Autodesk Inventor part; units mm, degrees
ref_plane "YZ Plane" through (0, 0, 0) normal (1, 0, 0) x (0, 1, 0)
ref_plane "XZ Plane" through (0, 0, 0) normal (0, 1, 0) x (-1, 0, 0)
ref_plane "XY Plane" through (0, 0, 0) normal (0, 0, 1) x (1, 0, 0)
sketch "スケッチ1" plane through (0, 0, 0) normal (0, 0, 1) x (1, 0, 0)
  line L0 (-12.5, -12.5) -> (12.5, -12.5) construction
  line L1 (12.5, -12.5) -> (12.5, 12.5) construction
  line L2 (12.5, 12.5) -> (-12.5, 12.5) construction
  line L3 (-12.5, 12.5) -> (-12.5, -12.5) construction
  line L4 (-12.5, -12.5) -> (12.5, 12.5) construction
  line L5 (12.5, -12.5) -> (-12.5, 12.5) construction
  line L6 (-8.1, 12.5) -> (-12.5, 12.5)
  line L7 (-12.5, 12.5) -> (-12.5, 8.1)
  line L8 (8.1, 12.5) -> (12.5, 12.5)
  line L9 (12.5, 12.5) -> (12.5, 8.1)
  line L10 (-12.5, -8.1) -> (-12.5, -12.5)
  line L11 (-12.5, -12.5) -> (-8.1, -12.5)
  line L12 (8.1, -12.5) -> (12.5, -12.5)
  line L13 (12.5, -12.5) -> (12.5, -8.1)
  line L14 (-6, 12.5) -> (-6, 14.5)
  line L15 (-6, 14.5) -> (6, 14.5)
  line L16 (6, 14.5) -> (6, 12.5)
  arc A0 (-8.1, 12.5) -> (-6, 12.5) centre (-7.05, 12.5) ccw
  arc A1 (6, 12.5) -> (8.1, 12.5) centre (7.05, 12.5) ccw
  line L17 (0, 12.5) -> (0, 0) construction
  line L18 (0, 0) -> (12.5, 0) construction
  line L19 (-12.5, 6) -> (-14.5, 6) construction
  line L20 (-14.5, 6) -> (-14.5, -6) construction
  line L21 (-14.5, -6) -> (-12.5, -6) construction
  arc A2 (-12.5, 6) -> (-12.5, 8.1) centre (-12.5, 7.05) ccw
  arc A3 (-12.5, -8.1) -> (-12.5, -6) centre (-12.5, -7.05) ccw construction
  line L22 (-6, -12.5) -> (-6, -14.5)
  line L23 (-6, -14.5) -> (6, -14.5)
  line L24 (6, -14.5) -> (6, -12.5)
  arc A4 (-6, -12.5) -> (-8.1, -12.5) centre (-7.05, -12.5) ccw
  arc A5 (8.1, -12.5) -> (6, -12.5) centre (7.05, -12.5) ccw
  line L25 (12.5, 6) -> (14.5, 6) construction
  line L26 (14.5, 6) -> (14.5, -6) construction
  line L27 (14.5, -6) -> (12.5, -6) construction
  arc A6 (12.5, 8.1) -> (12.5, 6) centre (12.5, 7.05) ccw construction
  arc A7 (12.5, -6) -> (12.5, -8.1) centre (12.5, -7.05) ccw construction
  line L28 (-9.05, 12.5) -> (-5.95, 12.5) construction
  line L29 (-5.95, 12.5) -> (-5.95, 9.5) construction
  line L30 (-5.95, 9.5) -> (-9.05, 9.5) construction
  line L31 (-9.05, 9.5) -> (-9.05, 12.5) construction
  line L32 (-12.5, 9.05) -> (-9.5, 9.05) construction
  line L33 (-9.5, 5.95) -> (-12.5, 5.95) construction
  line L34 (-12.5, 5.95) -> (-12.5, 9.05) construction
  line L35 (-7.5, 12.5) -> (-7.5, 9.5) construction
  line L36 (-9.5, 7.5) -> (-12.5, 7.5) construction
  line L37 (-12.5, -12.5) -> (-12.5, 12.5)
  line L38 (12.5, -12.5) -> (12.5, 12.5)
  dimension "d0" = 25
  dimension "d1" = 1.05
  dimension "d2" = 2
  dimension "d3" = 6.5
  dimension "d4" = 3.1
  dimension "d6" = 3
  dimension "d17" = 5
  dimension "d18" = 5
  dimension "d46" = 25
extrude "押し出し1" add sketch "スケッチ1" along normal blind 4
mirror "ミラー1" about plane through (0, 0, 0) normal (0, 0, -1) of "押し出し1"
sketch "スケッチ2" plane through (-12.5, -12.5, 4) normal (0, -1, 0) x (1, 0, 0)
  line L0 (6.5, 0) -> (18.5, 0) construction
  line L1 (12.5, 0) -> (12.5, -5) construction
  line L2 (0, -8) -> (0, 0) construction
  line L3 (0, -2.5) -> (22.3, -2.5) construction
  point P0 (12.5, -4)
  point P1 (2.7, -2.5)
  point P2 (0.0223, -2.5)
  dimension "d52" = 2.7
  dimension "d53" = 2.5
hole "穴1" at (-9.8, -12.5, 1.5) at (9.8, -12.5, 1.5) direction (0, 1, 0) diameter 2.459 depth 8.8
pattern_circular "円形状パターン1" count 2 over 360 about axis through (0, 0, -10) along (0, 0, 1) of "穴1"
sketch "スケッチ4" plane through (-8.1, -12.5, -4) normal (0, 0, -1) x (-1, 0, 0)
  circle A0 centre (-8.1, 4) radius 1.5
  line L0 (-8.1, 4) -> (-8.1, 12.5) construction
  circle A1 centre (0.4, 12.5) radius 1.5
  circle A2 centre (-8.1, 21) radius 1.5
  circle A3 centre (-16.6, 12.5) radius 1.5
  dimension "d35" = 3
  dimension "d36" = 8.5
  dimension "d39" = 360
extrude "押し出し3" cut sketch "スケッチ4" against normal through all
sketch "スケッチ5" plane through (-8.1, -12.5, -4) normal (0, 0, -1) x (-1, 0, 0)
  circle A0 centre (-8.1, 12.5) radius 5.05
  dimension "d43" = 10.1
extrude "押し出し4" cut sketch "スケッチ5" against normal blind 2
sketch "スケッチ6" plane through (0, 0, 4) normal (0, 0, 1) x (1, 0, 0)
  circle A0 centre (8.5, 0) radius 1.5 construction
  circle A1 centre (0, 8.5) radius 1.5 construction
  circle A2 centre (-8.5, 0) radius 1.5 construction
  circle A3 centre (0, -8.5) radius 1.5 construction
  line L0 (0, -8.5) -> (0, 8.5) construction
  line L1 (8.5, 0) -> (-8.5, 0) construction
  circle A4 centre (0, 0) radius 5.05
  dimension "d47" = 10.1
extrude "押し出し5" cut sketch "スケッチ6" against normal up to surface (8 mm away)
sketch "スケッチ8" plane through (6, 14.5, -4) normal (0, 0, -1) x (-1, 0, 0)
  line L0 (0, -29) -> (0, -27)
  line L1 (12, -29) -> (0, -29)
  line L2 (12, -27) -> (12, -29)
  line L3 (0, 0) -> (12, 0)
  line L4 (0, -2) -> (0, 0)
  line L5 (12, 0) -> (12, -2)
  line L6 (0, -27) -> (12, -27)
  line L7 (0, -2) -> (12, -2)
  point P0 (6, -14.5)
extrude "押し出し6" cut sketch "スケッチ8" against normal blind 3
equation "\"d18\" = d17"
properties part number "頭_サーボホーンフレーム" material "アセタール樹脂、黒"
Design review of the part built by this model. Coordinates are the model's own, in mm. A direction names the side the tool comes from. Coordinates: 2 decimals unless noted, no trailing zeros. Order: outer loops, then holes, each group sorted by start corner. A loop starts at its lowest first (then second) coordinate and runs counter-clockwise, first axis right, second up.
Item 1: The part is to be moulded in two halves that separate along Z. For faces 4 (the flat face through (-10, 3.7, 2)), 5 (the flat face through (-10, -3.7, 2)), 6 (the cylindrical face through (7.07, 11.45, -0.06)), 7 (the flat face through (0, 6, -4)), say which applies: pulls with the +Z half, pulls with the -Z half, needs draft (parallel to the pull), parting line crosses it, or undercut.
Item 2: Take a section at D-D, the plane y = 0. Write out the cut boundary in (x, z).
Item 3: For pin 1 Ø2 at (x, z) = (-9.8, 1.5) entering from +Y; pin 2 Ø2 at (x, z) = (11, -2) entering from +Y; pin 3 Ø5 at (x, y) = (0, 8.5) entering from +Z; pin 4 Ø1 at (y, z) = (14, 1) entering from +X, all flat-tipped, find the tip position at first contact; note any pin that passes through.
Item 4: For line 1 (X direction, y = -6, z = 1.5); line 2 (Y direction, x = -8.5, z = 1.75); line 3 (Y direction, x = 0, z = 0.75), list the stretches that pass through material, from the lowest coordinate up.
Item 5: Take a section at A-A, the plane y = -8.5. Write out the cut boundary in (x, z).
Item 6: Take a section at C-C, the plane x = 7.5. Write out the cut boundary in (y, z), then the cut area to 3 significant figures.
Item 7: For faces 1 (the flat face through (-6, 13, 1)), 2 (the flat face through (6, -14, 1)), 3 (the flat face through (10, 12.5, 0)), list the 3-axis set-ups (+Z, -Z, +X, -X, +Y, -Y) from which the entire face can be reached by the end or side of a thin tool; tool diameter is ignored.
Item 8: Take a section at B-B, the plane z = -1.5. Write out the cut boundary in (x, y), then the cut area to 3 significant figures.
The answers:
1. face 4: undercut
1. face 5: undercut
1. face 6: needs draft
1. face 7: pulls with the -Z half
2. outline: (-12.5, -4) - (-10, -4) - (-10, 4) - (-12.5, 4) - close; (-7, -4) - (-5.05, -4) - (-5.05, 4) - (-7, 4) - close; (5.05, -4) - (7, -4) - (7, 4) - (5.05, 4) - close; (10, -4) - (12.5, -4) - (12.5, 4) - (10, 4) - close
3. pin 1: stops at y = 3.7
3. pin 2: stops at y = 12.5
3. pin 3: stops at z = 4
3. pin 4: stops at x = 6
4. line 1: x = -12.5 to -11.03, -8.57 to 8.57, 11.03 to 12.5
4. line 2: y = -12.5 to -1.5, 1.5 to 12.5
4. line 3: y = -14.5 to -10, -7 to -5.05, 5.05 to 7, 10 to 14.5
5. outline: (-12.5, -4) - (-1.5, -4) - (-1.5, 4) - (-12.5, 4) - close; (1.5, -4) - (12.5, -4) - (12.5, 4) - (1.5, 4) - close; hole circle Ø2.46 at (-9.8, 1.5); hole circle Ø2.46 at (9.8, 1.5)
6. outline: (-11.55, -4) - (-1.12, -4) - (-1.12, 4) - (-11.55, 4) - close; (1.12, -4) - (11.55, -4) - (11.55, 4) - (1.12, 4) - close
6. area: 167 mm2
7. face 1: +Z, -Z, -X, +Y
7. face 2: +Z, -Z, +X, -Y
7. face 3: +Z, -Z, +X, +Y
8. outline: (-12.5, -12.5) - (-8.1, -12.5) arc R1.05 cw to (-6, -12.5) - (6, -12.5) arc R1.05 cw to (8.1, -12.5) - (12.5, -12.5) - (12.5, 12.5) - (8.1, 12.5) arc R1.05 cw to (6, 12.5) - (-6, 12.5) arc R1.05 cw to (-8.1, 12.5) - (-12.5, 12.5) - close; hole circle Ø3 at (-8.5, 0); hole circle Ø10.1 at (0, 0); hole circle Ø3 at (0, -8.5); hole circle Ø3 at (0, 8.5); hole circle Ø3 at (8.5, 0)
8. area: 510 mm2
